Geometry: see drawing. Coordinates: mm, zero at the bounding-box minimum. A direction names the side the tool comes from. Coordinates: 2 decimals unless noted, no trailing zeros. Write each loop counter-clockwise with the first axis right and the second up, starting at its lowest first coordinate (ties: lowest second). Pieces come first, ordered by that corner, then holes. Notation, with made-up numbers: (-17, 18.25) -> (-2, 18.25) arc R34 cw to (-2, 50.25) -> close; hole circle Ø8 at (29.5, 66.25). An arc over 180 degrees is marked (long way). Answer as a JSON object with one key per item and string values. Group by question number.
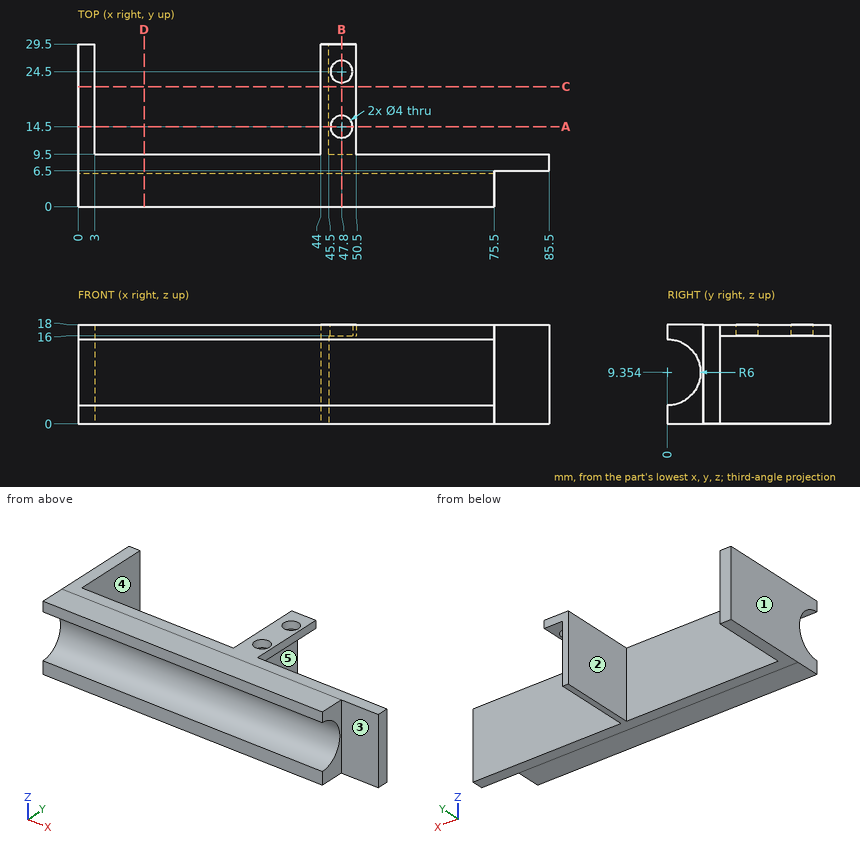
Item 1: Section A-A on y = 14.5. Output: boundary loops of the cut face in (x, z).
Item 2: Ray query, L1, parallel to Y at x = 47.8, z = 17.5; L2, parallel to X at y = 26.75, z = 13; L3, parallel to Y at x = 20, z = 1.25. Return the intervals inside material, ascending. Write a range as [from, to].
Item 3: Contact query for flat-ended pins moving along their axis: pin 1 (10 mm diameter, centred on x = 36, z = 14, fed in from +Y); pin 2 (5 mm diameter, centred on y = 2, z = 5.5, fed in from +X); pin 3 (4 mm diameter, centred on x = 48.5, y = 21.5, fed in from -Z). Output: stop coordinate, or through.
Item 4: Section D-D on x = 12. Output: boundary loops of the cut face in (y, z).
Item 5: Section B-B on x = 47.8. Output: boundary loops of the cut face in (y, z).
Item 6: Section C-C on y = 21.75. Output: boundary loops of the cut face in (x, z).
Item 7: Mould query, pull axis X, two halves, no side actions, for the marked faces 3, 4 and 5. Classes: +X half, -X half, draft (parallel to the pull), parting line (faces both ways), or undercut.
Item 8: Set-up query: the marked faces 1 and 2. Return all of +Z, -Z, +X, -X, +Y, -Y with unobstructed straight access to the full face (end or side cutting, diameter ignored); none if empty.
Answer sheet:
{
 "1": {"outline": "(0, 0) -> (3, 0) -> (3, 18) -> (0, 18) -> close; (44, 0) -> (45.5, 0) -> (45.5, 16) -> (45.8, 16) -> (45.8, 18) -> (44, 18) -> close; (49.8, 16) -> (50.5, 16) -> (50.5, 18) -> (49.8, 18) -> close"},
 "2": {"L1": "y = [0, 12.5], [16.5, 22.5], [26.5, 29.5]", "L2": "x = [0, 3], [44, 45.5]", "L3": "y = [0, 9.5]"},
 "3": {"pin 1": "stops at y = 9.5", "pin 2": "stops at x = 75.5", "pin 3": "stops at z = 16"},
 "4": {"outline": "(0, 0) -> (9.5, 0) -> (9.5, 18) -> (0, 18) -> (0, 15.35) arc R6 cw to (0, 3.35) -> close"},
 "5": {"outline": "(0, 0) -> (9.5, 0) -> (9.5, 16) -> (12.5, 16) -> (12.5, 18) -> (0, 18) -> (0, 15.35) arc R6 cw to (0, 3.35) -> close; (16.5, 16) -> (22.5, 16) -> (22.5, 18) -> (16.5, 18) -> close; (26.5, 16) -> (29.5, 16) -> (29.5, 18) -> (26.5, 18) -> close"},
 "6": {"outline": "(0, 0) -> (3, 0) -> (3, 18) -> (0, 18) -> close; (44, 0) -> (45.5, 0) -> (45.5, 16) -> (50.5, 16) -> (50.5, 18) -> (44, 18) -> close"},
 "7": {"face 3": "draft", "face 4": "undercut", "face 5": "+X half"},
 "8": {"face 1": "+Z, -Z, -X, +Y, -Y", "face 2": "+Z, -Z, +Y"}
}
